Source: three-view drawing plus pictorial views. Frame: mm from the lowest corner of the part. Give positions to 0.01 mm unless a question says otherwise; leave off trailing zeros. Write each loop counter-clockwise with the first axis right and the second up, starting at its lowest first coordinate (ties: lowest second). Pieces come first, ordered by that corner, then holes. Notation, with made-up numbers: (75, 52) -> (134, 52) arc R29 cw to (134, 86) -> close; hole circle Ø5 at (87, -17.5). An arc over 180 degrees is marked (long way). Use a Markdown table: item, result. Add a question column.
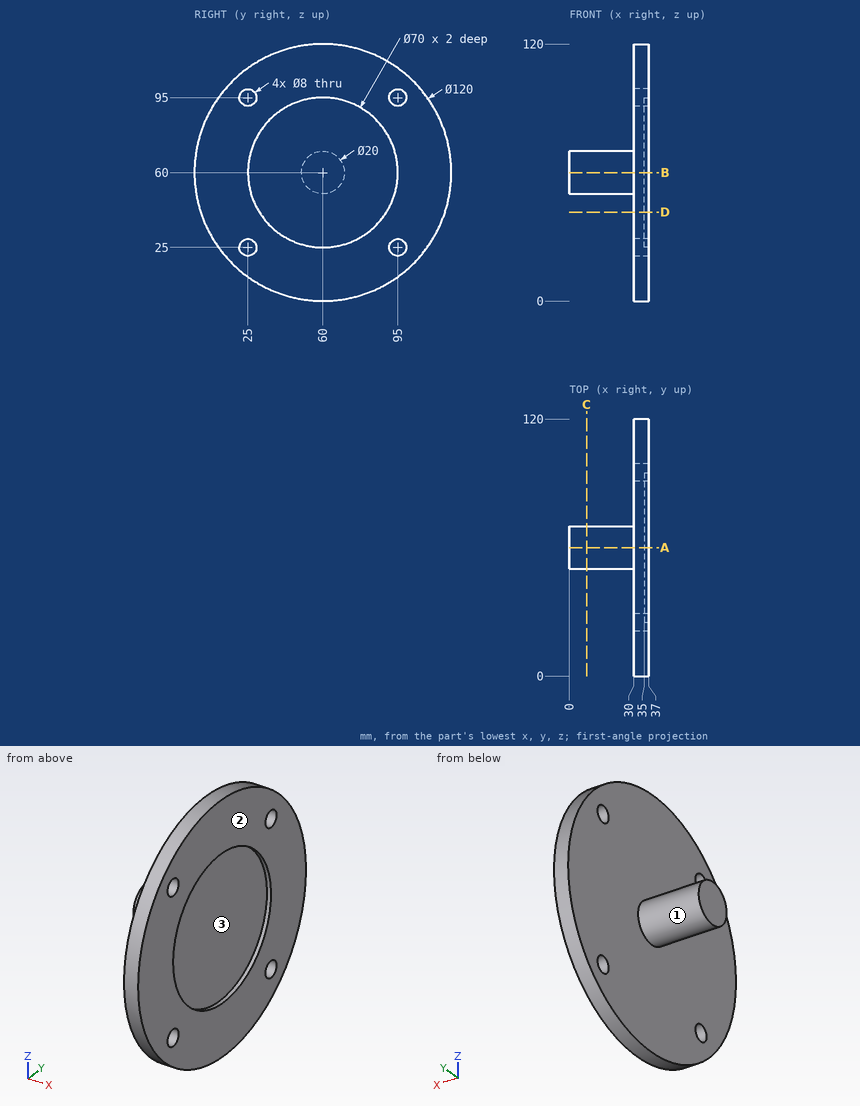
(1) Cut plane C-C on x = 8. Return the cut outline in (y, z), then the cut area to 3 significant figures.
(2) Cut plane D-D on z = 41.5. Return the cut outline in (x, y).
(3) Cut plane A-A on y = 60. Return the cut outline in (x, z).
(4) First-contact query: pin 1 Ø6 at (x, y) = (28, 100.5) entering from -Z; pin 2 Ø12 at (x, y) = (24.5, 55.5) entering from -Z; pin 3 Ø5 at (x, z) = (28, 62.5) entering from +Y; pin 4 Ø9 at (y, z) = (95, 95) entering from +X. Flat tips, straight axial feed; report the tip coordinate or a pass-through.
(5) Material intervals for L1, parallel to Y at x = 33.75, z = 95; L2, parallel to X at y = 79, z = 83, sorted ascending.
(6) Mould query, pull axis Y, two halves, no side actions, for the marked faces 1, 2 and 3. Classes: +Y half, -Y half, draft (parallel to the pull), parting line (faces both ways), or undercut.
Output:
| question | item | result |
|---|---|---|
| 1 | outline | circle Ø20 at (60, 60) |
| 1 | area | 314 mm^2 |
| 2 | outline | (30, 2.92) -> (37, 2.92) -> (37, 30.29) -> (35, 30.29) -> (35, 89.71) -> (37, 89.71) -> (37, 117.08) -> (30, 117.08) -> close |
| 3 | outline | (0, 50) -> (30, 50) -> (30, 0) -> (37, 0) -> (37, 25) -> (35, 25) -> (35, 95) -> (37, 95) -> (37, 120) -> (30, 120) -> (30, 70) -> (0, 70) -> close |
| 4 | pin 1 | z = 13.78 |
| 4 | pin 2 | z = 0.04 |
| 4 | pin 3 | y = 119.99 |
| 4 | pin 4 | x = 37 |
| 5 | L1 | 11.27 to 21, 29 to 91, 99 to 108.73 |
| 5 | L2 | 30 to 35 |
| 6 | face 1 | parting line |
| 6 | face 2 | draft |
| 6 | face 3 | undercut |
